Check sheet for the modelled part. Datum: model origin and axes. Units: mm. A direction names the side the tool comes from. Round coordinates to 2 decimals unless told otherwise and drop trailing zeros. Order: outer loops, then holes, each group sorted by start corner. A loop starts at its lowest first (then second) coordinate and runs counter-clockwise, first axis right, second up. Notation, with made-up numbers: M 75.25,39.5 L 103.25,39.5 A16 ccw 103.25,67.5 Z; hole C 23.5,31.5 d9. An arc over 180 degrees is marked long. One line per item, written item: value. Start each with the question number.
(1) Depth check by flat-ended pin: pin 1 Ø8 at (x, z) = (-3.5, 19.5) entering from +Y; pin 2 Ø1 at (y, z) = (-0.5, 15) entering from -X; pin 3 Ø1.5 at (x, z) = (-1, 8.5) entering from -Y. Enter the tip coordinate at first touch or a pass-through.
(2) Cross-section at C-C, the plane z = 14.25. Enter the section's corners in (x, y).
(3) Cross-section at B-B, the plane z = 22.5. Enter the section's corners in (x, y).
(4) Thickness scan on L1, parallel to Y at x = -2, z = 5; L2, parallel to X at y = 0, z = 3.95; L3, parallel to X at y = 0, z = 2.25. Record the ranges inside material, lowest first.
(5) Release check for a two-part mould opening along Y. For faces 3 (the face through (3.991, 0.022, 2.255)), 4 (the face through (-1.7, -4.3, 0)), 5 (the face through (5.416, 3.177, 3.827)) record: released by +Y, released by -Y, zero draft, split by the parting line, or undercut.
(6) Access from +Z, -Z, +X, -X, +Y, -Y to the whole of each face (thin tool, end or side, straight path). Record for faces 1 (the face through (4, 0, 0.4)), 2 (the face through (0, -4, 4.6)).
(7) Cross-section at A-A, the plane z = 7.25. Enter the section's corners in (x, y), and give its area (3 significant figures).
from build123d import *

# Parameters (mm, degrees)
SKETCH001_R         = 16.146195
POCKET_DEPTH        = 25.001
REVOLUTION001_ANGLE = 45
REVOLUTION002_ANGLE = 45


with BuildPart() as part:
    # Sketch → Revolution (revolve)
    with BuildSketch(Plane.XZ):
        Polygon((-1, 14.6), (-2.3, 14.6), (-3.2, 6.5), (-4.38, 5), (-4.38, 0), (-7, 0), (-7, 5), (-4.118425, 16.036616), (-2.121099, 17.791842), (-0.8, 25), (-0.6, 25), align=None)
    revolve(axis=Axis((0, 0, 0), (0, 0, 1)))

    # Sketch001 (on Face7 of Revolution) → Pocket (cut, through all)
    with BuildSketch(Plane(origin=(0, 0, 0), x_dir=(1, 0, 0), z_dir=(0, 0, -1))):
        Circle(SKETCH001_R)
        Polygon((-3.625, 6.278684), (-7.25, 0), (-3.625, -6.278684), (3.625, -6.278684), (7.25, 0), (3.625, 6.278684), align=None, mode=Mode.SUBTRACT)
    extrude(amount=-POCKET_DEPTH, mode=Mode.SUBTRACT)

    # Sketch002 → Revolution001 (revolve, symmetric)
    with BuildSketch(Plane.XZ) as revolution001_sk:
        Polygon((-4.88, 4.666667), (-4.38, 4.666667), (-3.75, 4), (-4.38, 3.333333), (-3.75, 2.666667), (-4.38, 2), (-3.75, 1.333333), (-4.38, 0.666667), (-4.88, 0.666667), align=None)
        Polygon((4.88, 0), (4.88, 4), (4.38, 4), (3.75, 3.333333), (4.38, 2.666667), (3.75, 2), (4.38, 1.333333), (3.75, 0.666667), (4.38, 0), align=None)
    revolve(axis=Axis((0, 0, 0), (0, 0, 1)), revolution_arc=REVOLUTION001_ANGLE / 2)
    revolve(revolution001_sk.sketch, axis=Axis((0, 0, 0), (0, 0, -1)), revolution_arc=REVOLUTION001_ANGLE / 2)

    # Sketch003 → Revolution002 (revolve, symmetric)
    with BuildSketch(Plane.YZ) as revolution002_sk:
        Polygon((-4.88, 5), (-4.38, 5), (-3.75, 4.333333), (-4.38, 3.666667), (-3.75, 3), (-4.38, 2.333333), (-3.75, 1.666667), (-4.38, 1), (-4.88, 1), align=None)
        Polygon((4.88, 0.333333), (4.88, 4.333333), (4.38, 4.333333), (3.75, 3.666667), (4.38, 3), (3.75, 2.333333), (4.38, 1.666667), (3.75, 1), (4.38, 0.333333), align=None)
    revolve(axis=Axis((0, 0, 0), (0, 0, 1)), revolution_arc=REVOLUTION002_ANGLE / 2)
    revolve(revolution002_sk.sketch, axis=Axis((0, 0, 0), (0, 0, -1)), revolution_arc=REVOLUTION002_ANGLE / 2)


solid = part.part
Values found:
1. pin 1: y = 3.84
1. pin 2: x = -4.5
1. pin 3: y = -6.23
2. outline: C 0,0 d9.17; hole C 0,0 d4.68
3. outline: C 0,0 d2.52; hole C 0,0 d1.39
4. L1: -6.28 to -3.9, 3.9 to 6.28
4. L2: -7 to -3.8, 4.33 to 7
4. L3: -7 to -4.14, 3.99 to 7
5. face 3: undercut
5. face 4: zero draft
5. face 5: released by +Y
6. face 1: -Z
6. face 2: none
7. outline: M -6.09,-2.01 L -4.79,-4.27 A6.41 ccw -1.3,-6.28 L 1.3,-6.28 A6.41 ccw 4.79,-4.27 L 6.09,-2.01 A6.41 ccw 6.09,2.01 L 4.79,4.27 A6.41 ccw 1.3,6.28 L -1.3,6.28 A6.41 ccw -4.79,4.27 L -6.09,2.01 A6.41 ccw Z; hole C 0,0 d6.23
7. area: 97.3 mm^2
